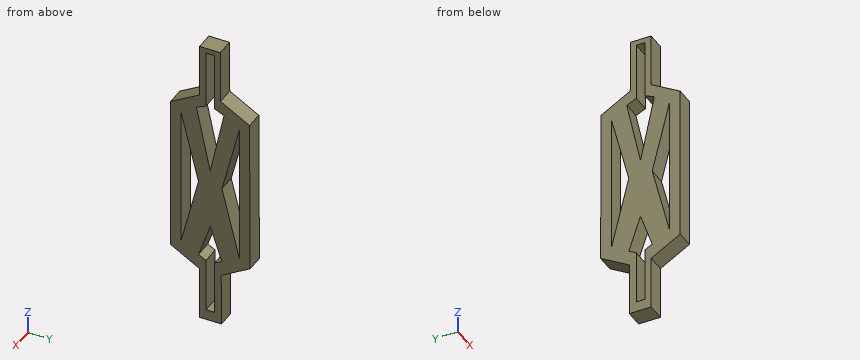
```python
from build123d import *

# Parameters (mm, degrees)
F1_DEPTH = 4
F2_DEPTH = 6


with BuildPart() as f1:
    # F0 (on Right) → F1 (new body)
    with BuildSketch(Plane.YZ):
        Polygon((3.420798, 50.363688), (-3.613221, 50.350249), (-3.613221, 32.27243), (-13.464639, 26.55225), (-13.464639, -26.587166), (-3.613221, -32.290113), (-3.613221, -50.367933), (3.805658, -50.353758), (3.73658, -32.27607), (13.566135, -26.535521), (13.363081, 26.603507), (3.489876, 32.286001), align=None)
        Polygon((-1.448536, -46.818957), (-1.448536, -28.4841), (-3.981812, -27.11692), (0, -15.432488), (3.981812, -27.11692), (1.448536, -28.4841), (1.448536, -46.818957), align=None, mode=Mode.SUBTRACT)
        Polygon((-9.887695, -23.929583), (-9.887695, 23.680427), (-3.981812, 0), align=None, mode=Mode.SUBTRACT)
        Polygon((3.981812, 0), (9.887695, 23.680427), (9.887695, -23.929583), align=None, mode=Mode.SUBTRACT)
        Polygon((-1.448536, 28.89285), (-1.448536, 48.621111), (1.448536, 48.621111), (1.448536, 28.89285), (4.687637, 27.380314), (0, 5.270754), (-4.687637, 27.380314), align=None, mode=Mode.SUBTRACT)
    extrude(amount=F1_DEPTH)

    # F0 (on Right) → F2 (join)
    with BuildSketch(Plane.YZ):
        Polygon((3.420798, 50.363688), (-3.613221, 50.350249), (-3.613221, 32.27243), (-13.464639, 26.55225), (-13.464639, -26.587166), (-3.613221, -32.290113), (-3.613221, -50.367933), (3.805658, -50.353758), (3.73658, -32.27607), (13.566135, -26.535521), (13.363081, 26.603507), (3.489876, 32.286001), align=None)
        Polygon((-1.448536, -46.818957), (-1.448536, -28.4841), (-3.981812, -27.11692), (0, -15.432488), (3.981812, -27.11692), (1.448536, -28.4841), (1.448536, -46.818957), align=None, mode=Mode.SUBTRACT)
        Polygon((-9.887695, -23.929583), (-9.887695, 23.680427), (-3.981812, 0), align=None, mode=Mode.SUBTRACT)
        Polygon((3.981812, 0), (9.887695, 23.680427), (9.887695, -23.929583), align=None, mode=Mode.SUBTRACT)
        Polygon((-1.448536, 28.89285), (-1.448536, 48.621111), (1.448536, 48.621111), (1.448536, 28.89285), (4.687637, 27.380314), (0, 5.270754), (-4.687637, 27.380314), align=None, mode=Mode.SUBTRACT)
    extrude(amount=F2_DEPTH)


solid = f1.part
```
Geometry check sheet. Reference: the model listing, model coordinates, mm. Coordinates: 2 decimals unless noted, no trailing zeros. Order: outer loops, then holes, each group sorted by start corner. A loop starts at its lowest first (then second) coordinate and runs counter-clockwise, first axis right, second up. Notation, with made-up numbers: (41.25, 89.25) - (59.25, 89.25) arc R8 cw to (59.25, 99.25) - close; hole circle Ø10 at (-13, 83.5). An arc over 180 degrees is marked (long way). Answer in a Markdown table with one row per item. Add a question column.
1. Section check C-C (z = 11.5). Enter the section's corners in (x, y), plus the area to 3 significant figures.
2. Section check D-D (z = -44). Enter the section's corners in (x, y), plus the area to 3 significant figures.
3. Section check A-A (x = 2.65). Give the number of separate pieces and of enclosed holes in the cut face, plus the area to 3 significant figures.
4. Section check B-B (y = 7.75). Enter the section's corners in (x, z), plus the area to 3 significant figures.
5. Material ranges on L1, parallel to Y at x = 1.55, z = -34; L2, parallel to Y at x = 3.9, z = -19; L3, parallel to Y at x = 4.25, z = 35, recorded low to high. Write a range as [from, to].
6. Gauge pin test, flat ends, axial feed: pin 1 Ø3 at (x, z) = (4.5, 30.5) entering from -Y; pin 2 Ø1.8 at (x, z) = (4, 44.5) entering from -Y; pin 3 Ø1 at (x, y) = (4, 5.5) entering from -Z. Record the tip position at first contact, or that the pin passes through.
Data:
| question | item | result |
|---|---|---|
| 1 | outline | (0, -13.46) - (6, -13.46) - (6, -9.89) - (0, -9.89) - close; (0, -6.85) - (6, -6.85) - (6, -1.32) - (0, -1.32) - close; (0, 1.32) - (6, 1.32) - (6, 6.85) - (0, 6.85) - close; (0, 9.89) - (6, 9.89) - (6, 13.42) - (0, 13.42) - close |
| 1 | area | 109 mm² |
| 2 | outline | (0, -3.61) - (6, -3.61) - (6, -1.45) - (0, -1.45) - close; (0, 1.45) - (6, 1.45) - (6, 3.78) - (0, 3.78) - close |
| 2 | area | 27.0 mm² |
| 3 | separate pieces | 1 |
| 3 | enclosed holes | 4 |
| 3 | area | 1,330 mm² |
| 4 | outline | (0, -29.93) - (6, -29.93) - (6, -15.27) - (0, -15.27) - close; (0, 15.11) - (6, 15.11) - (6, 29.83) - (0, 29.83) - close |
| 4 | area | 176 mm² |
| 5 | L1 | y = [-3.61, -1.45], [1.45, 3.74] |
| 5 | L2 | y = [-13.46, -9.89], [-8.67, -1.22], [1.22, 8.67], [9.89, 13.54] |
| 5 | L3 | y = [-3.61, -1.45], [1.45, 3.48] |
| 6 | pin 1 | stops at y = -9.25 |
| 6 | pin 2 | stops at y = -3.61 |
| 6 | pin 3 | stops at z = -31.54 |
